Autodesk Inventor part; units mm, degrees
ref_plane "YZ Plane" through (0, 0, 0) normal (1, 0, 0) x (0, 1, 0)
ref_plane "XZ Plane" through (0, 0, 0) normal (0, 1, 0) x (-1, 0, 0)
ref_plane "XY Plane" through (0, 0, 0) normal (0, 0, 1) x (1, 0, 0)
sketch "Эскиз1" plane through (0, 0, 0) normal (0, 1, 0) x (-1, 0, 0)
  circle A0 centre (0, 0) radius 10
  circle A1 centre (0, 0) radius 3.5
  circle A2 centre (0, 0) radius 2
  dimension "d0" = 20
  dimension "d1" = 7
  dimension "d2" = 4
extrude "Выдавливание1" add sketch "Эскиз1" against normal blind 20 contours A0 | A1 | A2
extrude "Выдавливание2" add sketch "Эскиз1" along normal blind 3 contours A1
extrude "Выдавливание3" add sketch "Эскиз1" along normal blind 10.5 contours A2
sketch "Эскиз2" plane through (0, 10.5, 0) normal (0, 1, 0) x (1, 0, 0)
  circle A0 centre (0, 0) radius 2
  circle A1 centre (0, 0) radius 2
  circle A2 centre (0, 0) radius 3.5
  line L0 (-3.1623, -1.5) -> (3.1623, -1.5)
  point P0 (0, 2)
  point P1 (0, 3.5)
  point P2 (1.3229, -1.5)
  point P3 (-1.3229, -1.5)
  dimension "d9" = 1.5
extrude "Выдавливание4" cut sketch "Эскиз2" against normal blind 7 contours L0 A0 picked at (0.3089, -1.5908)
sketch "Эскиз3" plane through (0, -20, 0) normal (0, -1, 0) x (1, 0, 0)
  line L0 (6.3804, -7.7) -> (-6.3804, -7.7)
  line L1 (-6.3804, -7.7) -> (-6.3804, 7.7)
  line L2 (-6.3804, 7.7) -> (6.3804, 7.7)
  line L3 (6.3804, 7.7) -> (6.3804, -7.7)
  circle A0 centre (0, 0) radius 10
  arc A1 (6.3804, -7.7) -> (6.3804, 7.7) centre (0, 0) ccw
  arc A2 (-6.3804, 7.7) -> (-6.3804, -7.7) centre (0, 0) ccw
  line L4 (5.3804, 0.25) -> (7.3804, 0.25)
  line L5 (7.3804, 0.25) -> (7.3804, -0.25)
  line L6 (7.3804, -0.25) -> (5.3804, -0.25)
  line L7 (5.3804, -0.25) -> (5.3804, 0.25)
  line L8 (5.3804, 0.25) -> (7.3804, -0.25) construction
  line L9 (0, -7.7) -> (0, 7.7) construction
  line L10 (-5.3804, 0.25) -> (-7.3804, 0.25)
  line L11 (-7.3804, 0.25) -> (-7.3804, -0.25)
  line L12 (-7.3804, -0.25) -> (-5.3804, -0.25)
  line L13 (-5.3804, -0.25) -> (-5.3804, 0.25)
  point P0 (6.3804, 0)
  point P1 (-6.3804, -7.7)
  dimension "d12" = 15.4
  dimension "d13" = 2
  dimension "d14" = 0.5
extrude "Выдавливание5" add sketch "Эскиз3" along normal blind 36 contours L6 L7 L4 L3 | L3 L4 L5 L6 | L12 L11 L10 L1 | L1 L10 L13 L12
extrude "Выдавливание6" add sketch "Эскиз3" along normal blind 32 contours L0 L1 L12 L13 L10 L2 L3 L4 L7 L6 | L3 L6 L5 L4 A0 | A0 L1 L10 L11 L12
sketch "Эскиз4" plane through (0, -52, 0) normal (0, -1, 0) x (1, 0, 0)
  circle A0 centre (0, 0) radius 2
  circle A1 centre (0, 0) radius 3.1
  dimension "d19" = 6.2
extrude "Выдавливание7" add sketch "Эскиз4" along normal blind 2.1 contours A0 | A1
sketch "Эскиз5" plane through (0, 0, 0) normal (0, 1, 0) x (1, 0, 0)
  circle A0 centre (0, 0) radius 10 construction
  line L0 (0, 10) -> (0, -10) construction
  circle A1 centre (0, 7.5) radius 1
  circle A2 centre (0, -7.5) radius 1
  dimension "d22" = 7.5
  dimension "d23" = 15
  dimension "d24" = 2
hole "Отверстие1" at (0, 0, 7.5) direction (0, -1, 0) diameter 2 depth 8 tip angle 118
hole "Отверстие2" at (0, 0, -7.5) direction (0, -1, 0) diameter 2 depth 8 tip angle 118
properties part number "motor20"
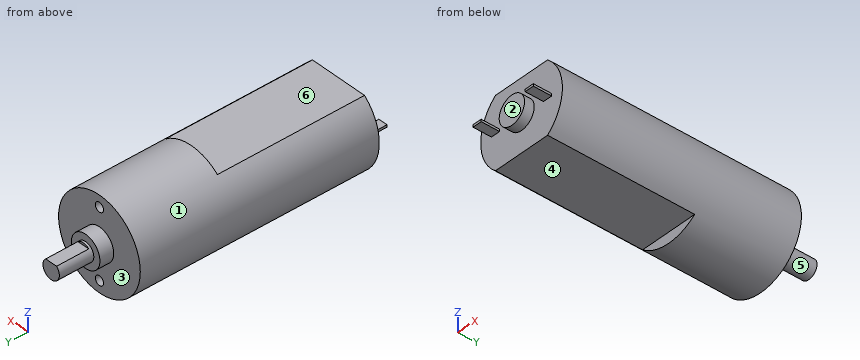
Check sheet for the modelled part. Datum: model origin and axes. Units: mm. Face numbers are marked on the shaded views. A direction names the side the tool comes from. Coordinates: 2 decimals unless noted, no trailing zeros. Loops run counter-clockwise (first coordinate to the right, second up) from the corner with the lowest first, then second, coordinate; pieces in that order, holes last. Notation, with made-up numbers: (-40, 6) -> (-33, 6) arc R19 cw to (-33, 23) -> close; hole circle Ø11 at (-33, 43). An arc over 180 degrees is marked (long way). Answer in a Markdown table with one row per item.
1. Sectioned sample at A-A, the plane y = -7. Record the boundary of the cut face in (x, z), then the cut area to 3 significant figures.
Check values:
| item | result |
|---|---|
| outline | circle Ø20 at (0, 0); hole circle Ø2 at (0, -7.5); hole circle Ø2 at (0, 7.5) |
| area | 308 mm2 |
2. Sectioned sample at B-B, the plane y = -29. Record the boundary of the cut face in (x, z).
Check values:
| item | result |
|---|---|
| outline | (-6.38, -7.7) -> (6.38, -7.7) arc R10 ccw to (6.38, 7.7) -> (-6.38, 7.7) arc R10 ccw to start |
3. Go/stop test with flat-tipped pins: pin 1 (1.6 mm diameter, centred on x = 6.5, y = -53.5, fed in from -Z); pin 2 (0.7 mm diameter, centred on x = 2.5, z = 9, fed in from -Y); pin 3 (1.9 mm diameter, centred on x = -1, z = 1.5, fed in from -Y). Record where each tip stops, or that it passes through.
Check values:
| item | result |
|---|---|
| pin 1 | stops at z = -0.25 |
| pin 2 | stops at y = -20 |
| pin 3 | stops at y = -54.1 |
4. Release check for a two-part mould opening along X. For the marked faces 1, 2 and 3 record: released by +X, released by -X, zero draft, split by the parting line, or undercut.
Check values:
| item | result |
|---|---|
| face 1 | split by the parting line |
| face 2 | undercut |
| face 3 | zero draft |
5. Access from +Z, -Z, +X, -X, +Y, -Y to the whole of each face (thin tool, end or side, straight path). Record for the marked faces 4, 5 and 6.
Check values:
| item | result |
|---|---|
| face 4 | -Z, +X, -X, -Y |
| face 5 | +Y |
| face 6 | +Z, +X, -X, -Y |
6. Material ranges on line 1 along Z through (x, y) = (0, -4.25); line 2 along Y through (x, z) = (-6, -7.5); line 3 along Z through (x, y) = (5.5, -26.5), recorded low to high. Write a range as [from, to].
Check values:
| item | result |
|---|---|
| line 1 | z = [-10, -8.5], [-6.5, 6.5], [8.5, 10] |
| line 2 | y = [-52, 0] |
| line 3 | z = [-7.7, 7.7] |
7. Sectioned sample at C-C, the plane z = 5.75. Record the boundary of the cut face in (x, y), then the cut area to 3 significant figures.
Check values:
| item | result |
|---|---|
| outline | (-8.18, -52) -> (8.18, -52) -> (8.18, 0) -> (-8.18, 0) -> close |
| area | 851 mm2 |
